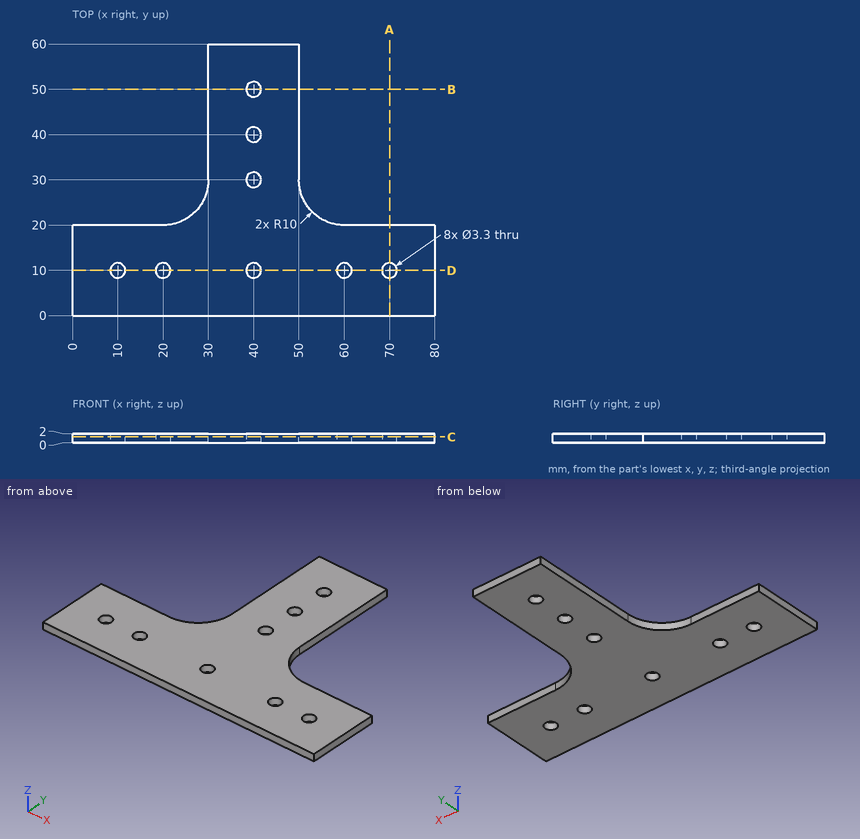
Geometry check sheet. Reference: drawing and pictorial views, mm from the part's lowest x, y, z. Round coordinates to 2 decimals unless told otherwise and drop trailing zeros. Loops run counter-clockwise (first coordinate to the right, second up) from the corner with the lowest first, then second, coordinate; pieces in that order, holes last.
1. Gauge pin test, flat ends, axial feed: pin 1 Ø3 at (x, y) = (40, 10) entering from -Z; pin 2 Ø0.6 at (x, z) = (74.5, 1.5) entering from +Y. Record the tip position at first contact, or that the pin passes through.
2. Sectioned sample at C-C on z = 1.3. Give the number of separate pieces and of enclosed holes in the cut face, and give its area (3 significant figures).
3. Sectioned sample at D-D on y = 10. Record the boundary of the cut face in (x, z), and give its area (3 significant figures).
4. Sectioned sample at A-A on x = 70. Record the boundary of the cut face in (y, z), and give its area (3 significant figures).
5. Scan lines: probe 1 along Y at (x, z) = (40, 0.55); probe 2 along Y at (x, z) = (60, 1.8); probe 3 along Y at (x, z) = (73, 0.95). Record each from-to range of solid material in increasing order.
6. Sectioned sample at B-B on y = 50. Record the boundary of the cut face in (x, z), and give its area (3 significant figures).
Recorded:
1. pin 1: passes through
1. pin 2: stops at y = 20
2. separate pieces: 1
2. enclosed holes: 8
2. area: 2,370 mm2
3. outline: (0, 0) - (8.35, 0) - (8.35, 2) - (0, 2) - close; (11.65, 0) - (18.35, 0) - (18.35, 2) - (11.65, 2) - close; (21.65, 0) - (38.35, 0) - (38.35, 2) - (21.65, 2) - close; (41.65, 0) - (58.35, 0) - (58.35, 2) - (41.65, 2) - close; (61.65, 0) - (68.35, 0) - (68.35, 2) - (61.65, 2) - close; (71.65, 0) - (80, 0) - (80, 2) - (71.65, 2) - close
3. area: 127 mm2
4. outline: (0, 0) - (8.35, 0) - (8.35, 2) - (0, 2) - close; (11.65, 0) - (20, 0) - (20, 2) - (11.65, 2) - close
4. area: 33.4 mm2
5. probe 1: y = 0 to 8.35, 11.65 to 28.35, 31.65 to 38.35, 41.65 to 48.35, 51.65 to 60
5. probe 2: y = 0 to 8.35, 11.65 to 20
5. probe 3: y = 0 to 20
6. outline: (30, 0) - (38.35, 0) - (38.35, 2) - (30, 2) - close; (41.65, 0) - (50, 0) - (50, 2) - (41.65, 2) - close
6. area: 33.4 mm2
